Geometry check sheet. Reference: the model listing, model coordinates, mm. A direction names the side the tool comes from. Round coordinates to 2 decimals unless told otherwise and drop trailing zeros. Order: outer loops, then holes, each group sorted by start corner. A loop starts at its lowest first (then second) coordinate and runs counter-clockwise, first axis right, second up.
(1) Sectioned sample at C-C (x = 20). Record the boundary of the cut face in (y, z).
(2) Release check for a two-part mould opening along Y. For faces 1 (the face through (4, 5, 5)), 2 (the face through (0, -22.5, 7)), 3 (the face through (22.5, 0, 27)) record: +Y half, -Y half, draft (parallel to the pull), parting line (faces both ways), or undercut.
(3) Sectioned sample at D-D (x = -16). Record the boundary of the cut face in (y, z).
(4) Set-up check for faces 4 (the face through (-2.17, -9.76, 7.43)), 5 (the face through (-0.2, 10.3, 9.8)), 6 (the face through (0, -21.5, -1)), 7 (the face through (-20.5, -2, 29)): record each of +Z, -Z, +X, -X, +Y, -Y from which the full face is reachable in a straight line by a thin tool's end or side.
(5) Go/stop test with flat-tipped pins: pin 1 (14.5 mm diameter, centred on y = 0, z = 33, fed in from -X); pin 2 (12 mm diameter, centred on x = 17, y = -6.5, fed in from -Z); pin 3 (1.1 mm diameter, centred on y = 22, z = -1, fed in from -X). Record where each tip stops, or that it passes through.
(6) Sectioned sample at A-A (x = 0). Record the boundary of the cut face in (y, z), plus the area to 3 significant figures.
(7) Sectioned sample at B-B (z = 13.5). Record the boundary of the cut face in (x, y), plus the area to 3 significant figures.
(8) Material ranges on line 1 along Y through (x, z) = (-17.8, 33); line 2 along Y through (x, z) = (0, 3); line 3 along X through (y, z) = (8, 39), recorded low to high.
from build123d import *

# Parameters (mm, degrees)
SKETCH_1_W          = 45
SKETCH_1_H          = 45
EXTRUDE_1_DEPTH     = 9.8
SKETCH_2_W          = 5.7
SKETCH_2_H          = 45
EXTRUDE_2_DEPTH     = 45.7
CUT_EXTRUDE_START   = -45
CUT_EXTRUDE_2_DEPTH = 45
SKETCH_4_R          = 4
CUT_EXTRUDE_3_DEPTH = 75.909945935
SKETCH_5_R          = 8
CUT_EXTRUDE_4_DEPTH = 2
SKETCH_6_R          = 6.1
CUT_EXTRUDE_5_DEPTH = 56.686533381
SKETCH_7_W          = 8.2
SKETCH_7_H          = 1
EXTRUDE_3_DEPTH     = 2
SKETCH_8_R          = 10
CUT_EXTRUDE_6_DEPTH = 4.8


# Read off the part's stored shape, not the designer's step: 切除-拉伸2
with BuildPart() as part:
    # 草图1 → 凸台-拉伸1 (new body)
    with BuildSketch(Plane.XY):
        Rectangle(SKETCH_1_W, SKETCH_1_H)
    extrude(amount=EXTRUDE_1_DEPTH)

    # 草图2 → 凸台-拉伸2 (add)
    with BuildSketch(Plane.XY.offset(9.8)):
        with Locations((-19.65, 0)):
            Rectangle(SKETCH_2_W, SKETCH_2_H)
        with Locations((19.65, 0)):
            Rectangle(SKETCH_2_W, SKETCH_2_H)
    extrude(amount=EXTRUDE_2_DEPTH)

    # 切除-拉伸2 outline → 切除-拉伸2 (cut)
    with BuildSketch(Plane.ZY.offset(22.5).offset(CUT_EXTRUDE_START)):
        with BuildLine():
            Line((55.5, 22.5), (33, 22.5))
            ThreePointArc((33, 22.5), (48.909902577, 15.909902577), (55.5, 0))
            Line((55.5, 0), (55.5, 22.5))
        make_face()
        with BuildLine():
            Line((55.5, -22.5), (55.5, 0))
            ThreePointArc((55.5, 0), (48.909902577, -15.909902577), (33, -22.5))
            Line((33, -22.5), (55.5, -22.5))
        make_face()
    extrude(amount=CUT_EXTRUDE_2_DEPTH, mode=Mode.SUBTRACT)

    # 草图4 → 切除-拉伸3 (cut, through all)
    with BuildSketch(Plane.ZY.offset(22.5)):
        with Locations((33, 0)):
            Circle(SKETCH_4_R)
    extrude(amount=-CUT_EXTRUDE_3_DEPTH, mode=Mode.SUBTRACT)

    # 草图5 → 切除-拉伸4 (cut)
    with BuildSketch(Plane.ZY.offset(22.5)):
        with Locations((33, 0)):
            Circle(SKETCH_5_R)
    extrude(amount=-CUT_EXTRUDE_4_DEPTH, mode=Mode.SUBTRACT)

    # 草图6 → 切除-拉伸5 (cut, through all)
    with BuildSketch(Plane.XY.offset(9.8)):
        Circle(SKETCH_6_R)
    extrude(amount=-CUT_EXTRUDE_5_DEPTH, mode=Mode.SUBTRACT)

    # 草图7 → 凸台-拉伸3 (add)
    with BuildSketch(Plane(origin=(0, 0, 0), x_dir=(-1, 0, 0), z_dir=(0, 0, -1))):
        with Locations((0, 22)):
            Rectangle(SKETCH_7_W, SKETCH_7_H)
        with Locations((0, -22)):
            Rectangle(SKETCH_7_W, SKETCH_7_H)
    extrude(amount=EXTRUDE_3_DEPTH)

    # 草图8 → 切除-拉伸6 (cut)
    with BuildSketch(Plane.XY.offset(9.8)):
        Circle(SKETCH_8_R)
    extrude(amount=-CUT_EXTRUDE_6_DEPTH, mode=Mode.SUBTRACT)


solid = part.part
Answer below:
1. outline: (-22.5, 0) - (22.5, 0) - (22.5, 33) arc R22.5 ccw to (-22.5, 33) - close; hole circle Ø8 at (0, 33)
2. face 1: undercut
2. face 2: -Y half
2. face 3: draft
3. outline: (-22.5, 0) - (22.5, 0) - (22.5, 9.8) - (-22.5, 9.8) - close
4. face 4: +Z
4. face 5: +Z, +Y, -Y
4. face 6: -Z, +X, -X
4. face 7: -X
5. pin 1: stops at x = -20.5
5. pin 2: stops at z = 0
5. pin 3: stops at x = -4.1
6. outline: (-22.5, -2) - (-21.5, -2) - (-21.5, 0) - (-6.1, 0) - (-6.1, 5) - (-10, 5) - (-10, 9.8) - (-22.5, 9.8) - close; (6.1, 0) - (21.5, 0) - (21.5, -2) - (22.5, -2) - (22.5, 9.8) - (10, 9.8) - (10, 5) - (6.1, 5) - close
6. area: 288 mm2
7. outline: (-22.5, -22.5) - (-16.8, -22.5) - (-16.8, 22.5) - (-22.5, 22.5) - close; (16.8, -22.5) - (22.5, -22.5) - (22.5, 22.5) - (16.8, 22.5) - close
7. area: 513 mm2
8. line 1: y = -22.5 to -4, 4 to 22.5
8. line 2: y = -22.5 to -6.1, 6.1 to 22.5
8. line 3: x = -22.5 to -16.8, 16.8 to 22.5
